Check sheet for the modelled part. Datum: model origin and axes. Units: mm. A direction names the side the tool comes from. Give positions to 0.01 mm unless a question says otherwise; leave off trailing zeros. Order: outer loops, then holes, each group sorted by start corner. A loop starts at its lowest first (then second) coordinate and runs counter-clockwise, first axis right, second up.
Autodesk Inventor part; units mm, degrees
ref_plane "YZ Plane" through (0, 0, 0) normal (1, 0, 0) x (0, 1, 0)
ref_plane "XZ Plane" through (0, 0, 0) normal (0, 1, 0) x (-1, 0, 0)
ref_plane "XY Plane" through (0, 0, 0) normal (0, 0, 1) x (1, 0, 0)
sketch "Skizze1" plane through (0, 0, 0) normal (1, 0, 0) x (0, 1, 0)
  line L0 (-19.25, -13.25) -> (19.25, -13.25)
  line L1 (19.25, -13.25) -> (19.25, 13.25)
  line L2 (19.25, 13.25) -> (-19.25, 13.25)
  line L3 (-19.25, 13.25) -> (-19.25, -13.25)
  line L4 (-19.25, -13.25) -> (19.25, 13.25) construction
  line L5 (19.25, -13.25) -> (-19.25, 13.25) construction
  point P0 (0, 0)
  dimension "d0" = 38.5
  dimension "d1" = 26.5
extrude "Extrusion1" add sketch "Skizze1" along normal blind 33
sketch "Skizze2" plane through (0, -19.25, 13.25) normal (0, 0, 1) x (1, 0, 0)
  line L0 (0, 38.5) -> (33, 38.5)
  line L1 (3, 38.5) -> (33, 38.5)
  line L2 (33, 38.5) -> (33, 3)
  line L3 (33, 3) -> (3, 3)
  line L4 (3, 3) -> (3, 38.5)
  point P0 (0, 19.25)
  dimension "d4" = 35.5
extrude "Extrusion2" cut sketch "Skizze2" against normal through all
sketch "Skizze3" plane through (0, 0, 0) normal (-1, 0, 0) x (0, 0, 1)
  line L0 (13.25, -16.25) -> (-13.25, -16.25)
  point P0 (0, 0)
  point P1 (0, 0.75)
  dimension "d14" = 0
  dimension "d15" = 17
hole "Bohrung1" at (0, 0.75, 0) direction (1, 0, 0) diameter 8 end through all
properties part number "MotorHalterNeu"
(1) Release check for a two-part mould opening along Y. For faces 1 (the face through (0, -5, 0)), 2 (the face through (18, -16.25, 0)), 3 (the face through (1.521, 4.655, -0.867)) record: released by +Y, released by -Y, zero draft, split by the parting line, or undercut.
Response values:
face 1: zero draft
face 2: released by +Y
face 3: undercut
(2) Cross-section at A-A on y = 0.75. Enter the section's corners in (x, z), then the cut area to 3 significant figures.
Response values:
outline: (0, -13.25) - (3, -13.25) - (3, -4) - (0, -4) - close; (0, 4) - (3, 4) - (3, 13.25) - (0, 13.25) - close
area: 55.5 mm2
(3) Cross-section at C-C on x = 13. Enter the section's corners in (y, z).
Response values:
outline: (-19.25, -13.25) - (-16.25, -13.25) - (-16.25, 13.25) - (-19.25, 13.25) - close
(4) Cross-section at B-B on z = 0. Enter the section's corners in (x, y), then the cut area to 4 significant figures.
Response values:
outline: (0, -19.25) - (33, -19.25) - (33, -16.25) - (3, -16.25) - (3, -3.25) - (0, -3.25) - close; (0, 4.75) - (3, 4.75) - (3, 19.25) - (0, 19.25) - close
area: 181.5 mm2
(5) Cross-section at D-D on z = 4.5. Enter the section's corners in (x, y), then the cut area to 4 significant figures.
Response values:
outline: (0, -19.25) - (33, -19.25) - (33, -16.25) - (3, -16.25) - (3, 19.25) - (0, 19.25) - close
area: 205.5 mm2
(6) Material ranges on L1, parallel to Z at x = 1.3, y = 0.75; L2, parallel to Y at x = 1.25, z = 0; L3, parallel to X at y = 14, z = 3, recorded low to high.
Response values:
L1: z = -13.25 to -4, 4 to 13.25
L2: y = -19.25 to -3.25, 4.75 to 19.25
L3: x = 0 to 3
(7) Gauge pin test, flat ends, axial feed: pin 1 Ø10.5 at (y, z) = (0.75, 0) entering from +X; pin 2 Ø8 at (x, z) = (13.5, -4.5) entering from +Y. Record the tip position at first contact, or that the pin passes through.
Response values:
pin 1: stops at x = 3
pin 2: stops at y = -16.25
(8) Set-up check for faces 4 (the face through (3, 5, 0)), 5 (the face through (33, -18, 0)): record each of +Z, -Z, +X, -X, +Y, -Y from which the full face is reachable in a straight line by a thin tool's end or side.
Response values:
face 4: +Z, -Z, +X, +Y
face 5: +Z, -Z, +X, +Y, -Y
